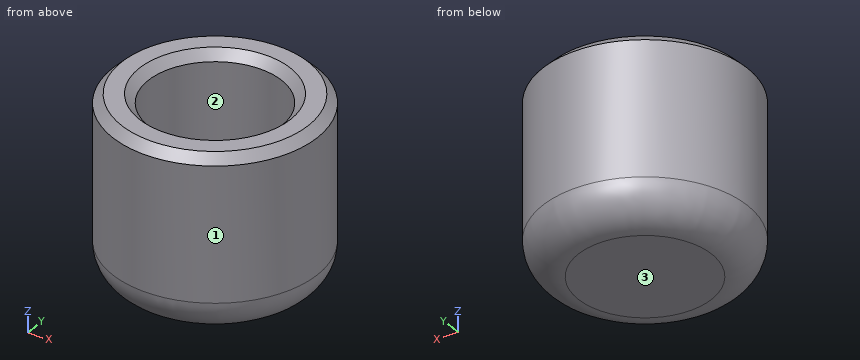
from build123d import *

# Parameters (mm, degrees)
F0_R     = 18.2245
F1_DEPTH = 31.75
F2_T     = -6.35
F3_R     = 6.35
F4_SIZE  = 1.5875


with BuildPart() as f1:
    # F0 (on Top) → F1 (new body)
    with BuildSketch(Plane.XY):
        Circle(F0_R)
    extrude(amount=F1_DEPTH)

    # F2
    f2_openings = [f1.faces().sort_by_distance(p)[0] for p in [
        (0, 0, 31.75),
    ]]
    offset(amount=F2_T, openings=f2_openings)

    # F3
    f3_edges = [f1.edges().sort_by_distance(p)[0] for p in [
        (-18.2245, 0, 0),
    ]]
    fillet(f3_edges, radius=F3_R)

    # F4
    f4_edges = [f1.edges().sort_by_distance(p)[0] for p in [
        (-18.2245, 0, 31.75),
        (-11.8745, 0, 31.75),
    ]]
    chamfer(f4_edges, length=F4_SIZE)


solid = f1.part
The model under review builds one solid part; all positions refer to its coordinate system, in mm. Face numbers are marked on the shaded views. Round coordinates to 2 decimals unless told otherwise and drop trailing zeros. Loops run counter-clockwise (first coordinate to the right, second up) from the corner with the lowest first, then second, coordinate; pieces in that order, holes last. Notation, with made-up numbers: M 10.5,-25 L 18.5,-25 A31 cw 18.5,-1 Z; hole C -35,35 d6. An arc over 180 degrees is marked long. Answer as CSV lines item,"result".
1. Insertion check: pin 1 Ø8 at (x, z) = (-5, 19) entering from -Y; pin 2 Ø14 at (x, y) = (0, 0) entering from +Z; pin 3 Ø8 at (x, z) = (3.5, 12) entering from +Y. Each pin has a flat end and moves straight along its axis. Give the tip position at first contact, or say it passes through.
Outcome:
pin 1,"stops at y = -18.2"
pin 2,"stops at z = 6.35"
pin 3,"stops at y = 18.22"
2. To check wall thickness, follow L1, parallel to Y at x = 0, z = 20; L2, parallel to Z at x = -6.5, y = 1; L3, parallel to X at y = -7, z = 22.5. State the ranges of each line that lie inside material, in increasing order. Write a range as [from, to].
Outcome:
L1,"y = [-18.22, -11.87], [11.87, 18.22]"
L2,"z = [0, 6.35]"
L3,"x = [-16.83, -9.59], [9.59, 16.83]"
3. Draft analysis for pull direction Y (two halves, no side actions). For the marked faces 1, 2 and 3, state which applies: pulls with the +Y half, pulls with the -Y half, needs draft (parallel to the pull), parting line crosses it, or undercut.
Outcome:
face 1,"parting line crosses it"
face 2,"undercut"
face 3,"needs draft"
4. We need section D-D (z = 5). Give the boundary of the cut face in (x, y), plus the area to 3 significant figures.
Outcome:
outline,"C 0,0 d36.16"
area,"1,030 mm2"
5. We need section C-C (z = 24.5). Give the boundary of the cut face in (x, y), plus the area to 3 significant figures.
Outcome:
outline,"C 0,0 d36.45; hole C 0,0 d23.75"
area,"600 mm2"
6. We need section A-A (x = 0). Give the boundary of the cut face in (y, z).
Outcome:
outline,"M -18.22,6.35 A6.35 ccw -11.87,0 L 11.87,0 A6.35 ccw 18.22,6.35 L 18.22,30.16 L 16.64,31.75 L 13.46,31.75 L 11.87,30.16 L 11.87,6.35 L -11.87,6.35 L -11.87,30.16 L -13.46,31.75 L -16.64,31.75 L -18.22,30.16 Z"
